The figure shows three views and two pictorial views of one solid part (mm, origin at its lowest corner). Answer the questions. A direction names the side the tool comes from. Coordinates: 2 decimals unless noted, no trailing zeros. Write each loop counter-clockwise with the first axis right and the second up, starting at its lowest first coordinate (ties: lowest second). Pieces come first, ordered by that corner, then holes. Notation, with made-up numbers: M 7,21.5 L 25,21.5 A8 ccw 25,36.5 Z; hole C 1.5,-37 d4. An arc over 180 degrees is marked long. Use CSV: the item, a comma, the result in double quotes.
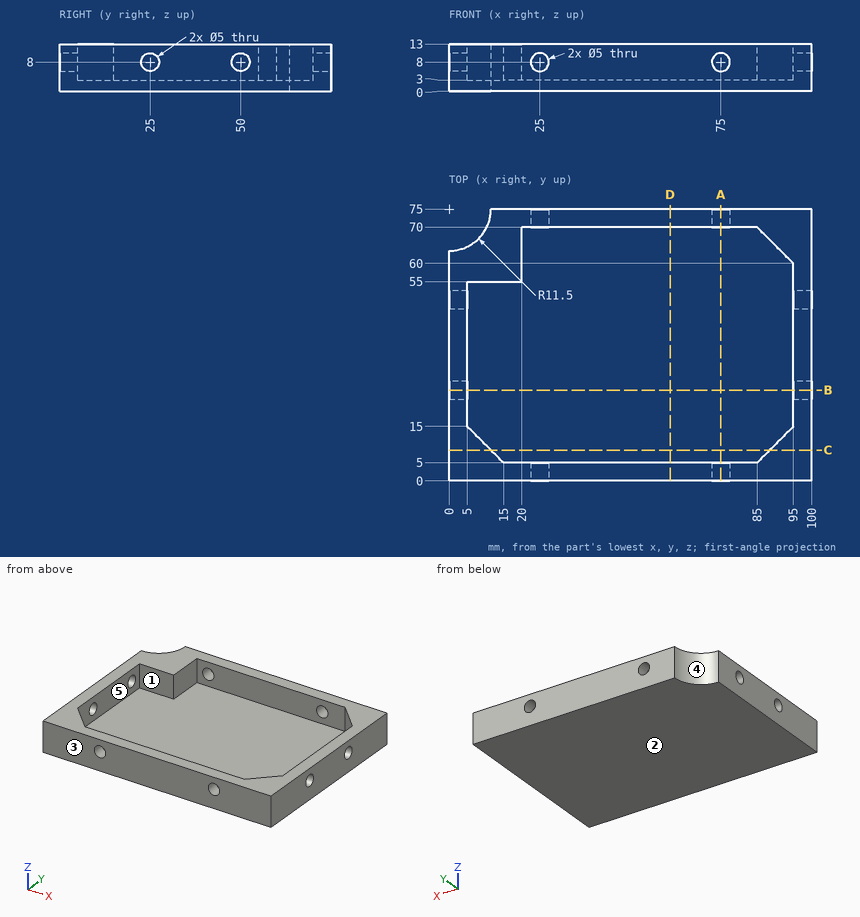
Item 1: The part is cut by section A-A (x = 75). Write down the section's boundary in (y, z).
Answer:
outline,"M 0,0 L 75,0 L 75,5.5 L 70,5.5 L 70,3 L 5,3 L 5,5.5 L 0,5.5 Z; M 0,10.5 L 5,10.5 L 5,13 L 0,13 Z; M 70,10.5 L 75,10.5 L 75,13 L 70,13 Z"
Item 2: The part is cut by section B-B (y = 25). Write down the section's boundary in (x, z).
Answer:
outline,"M 0,0 L 100,0 L 100,5.5 L 95,5.5 L 95,3 L 5,3 L 5,5.5 L 0,5.5 Z; M 0,10.5 L 5,10.5 L 5,13 L 0,13 Z; M 95,10.5 L 100,10.5 L 100,13 L 95,13 Z"
Item 3: A tool of negligible diameter and unlimited length cuts with its end or side. For the marked faces 4 and 5, from which of +Z, -Z, +X, -X, +Y, -Y can it reach the whole face along a straight path? Write none if from no direction.
Answer:
face 4,"+Z, -Z, -X, +Y"
face 5,"+Z"
Item 4: For a pull along Y with two mould halves and no side action, classify the marked faces 1, 2 and 3 as released by +Y, released by -Y, zero draft, split by the parting line, or undercut.
Answer:
face 1,"undercut"
face 2,"zero draft"
face 3,"released by -Y"
Item 5: The part is cut by section C-C (y = 8.5). Write down the section's boundary in (x, z), then the cut area to 3 significant figures.
Answer:
outline,"M 0,0 L 100,0 L 100,13 L 88.5,13 L 88.5,3 L 11.5,3 L 11.5,13 L 0,13 Z"
area,"530 mm2"
Item 6: Consider probe 1 along Y at (x, z) = (59, 10); probe 2 along Z at (x, y) = (96, 25); probe 3 along X at (y, z) = (26, 11). Determine where each line is inside the solid, lowest interval first.
Answer:
probe 1,"y = 0 to 5, 70 to 75"
probe 2,"z = 0 to 5.5, 10.5 to 13"
probe 3,"x = 0 to 5, 95 to 100"
Item 7: The part is cut by section D-D (x = 61). Write down the section's boundary in (y, z).
Answer:
outline,"M 0,0 L 75,0 L 75,13 L 70,13 L 70,3 L 5,3 L 5,13 L 0,13 Z"
Item 8: Given pin 1 (12 mm diameter, centred on x = 65, y = 16, fed in from +Z), flat-ended and moving along its own axis, determine where the tip first touches the part or whether it passes through.
Answer:
pin 1,"stops at z = 3"
